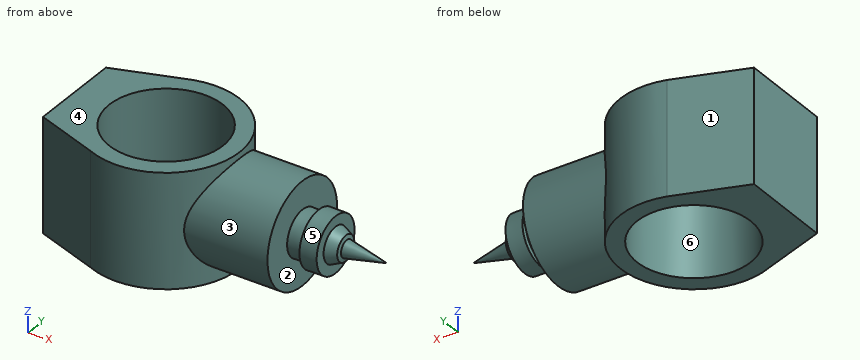
```python
from build123d import *

# Parameters (mm, degrees)
SKETCH1_R                = 50
BOSS_EXTRUDE1_DEPTH      = 50
BOSS_EXTRUDE2_REACH      = 218.485
BOSS_EXTRUDE2_END_RADIUS = 65
SKETCH2_R                = 45


with BuildPart() as part:
    # Sketch1 → Boss-Extrude1 (new, symmetric)
    with BuildSketch(Plane.XY):
        with BuildLine():
            Line((-80.332774103, 40.816671374), (-18.32732241, 62.420380787))
            ThreePointArc((-18.32732241, 62.420380787), (64.887320327, -3.869658553), (-25.718765207, -59.633296758))
            Line((-25.718765207, -59.633296758), (-80.331207523, -40.594442176))
            Line((-80.331207523, -40.594442176), (-80.332774103, 40.816671374))
        make_face()
        with Locations(Location((0.059475093, 0.33297887, 0), (0, 0, 180))):
            Circle(SKETCH1_R, mode=Mode.SUBTRACT)
    extrude(amount=BOSS_EXTRUDE1_DEPTH, both=True)

    # Boss-Extrude2: up to this cylinder (the profile starts outside it)
    boss_extrude2_end = Plane(origin=(0.006183555, 0.059475093, -0.380635), z_dir=(0, 0, -1)) * Cylinder(BOSS_EXTRUDE2_END_RADIUS, 567.97, mode=Mode.PRIVATE)
    # Sketch2 → Boss-Extrude2 (add, up to the surface)
    with BuildSketch(Plane(origin=(120, 0, 0), x_dir=(0, 0, -1), z_dir=(1, 0, 0)), mode=Mode.PRIVATE) as boss_extrude2_sk1:
        with Locations((0.380634668, -0.130842241)):
            Circle(SKETCH2_R)
    boss_extrude2_tool1 = extrude(boss_extrude2_sk1.sketch, amount=-BOSS_EXTRUDE2_REACH, mode=Mode.PRIVATE) - boss_extrude2_end
    add(boss_extrude2_tool1.solids().sort_by_distance((120, -0.130842, -0.380635))[0])

    # Sketch4 → Revolve1 (revolve)
    with BuildSketch(Plane.XY):
        Polygon((119.999333132, 0.283284997), (194.173107585, 0.294264183), (158.779171315, -7.089790216), (157.928859049, -10.799864107), (148.89148066, -15.080727554), (148.998076603, -24.232348433), (133.998076603, -24.369382261), (133.994271745, -19.369382261), (119.994271745, -19.700497331), align=None)
    revolve(axis=Axis((119.999333132, 0.283284997, 0), (0.9999999890450703, 0.00014801979444003187, 0)))


solid = part.part
```
The listing builds one solid part. Answer for the finished solid, in the listing's coordinates (mm). Face numbers are marked on the shaded views. A direction names the side the tool comes from. Round coordinates to 2 decimals unless told otherwise and drop trailing zeros. Order: outer loops, then holes, each group sorted by start corner. A loop starts at its lowest first (then second) coordinate and runs counter-clockwise, first axis right, second up. Notation, with made-up numbers: (61.25, 32.25) -> (65.25, 32.25) arc R20 ccw to (65.25, 64.25) -> close; hole circle Ø7 at (-13.5, 15.25). An arc over 180 degrees is marked (long way). Answer as CSV lines item,"result".
Q1. Consider line 1 (X direction, y = 0, z = 17); line 2 (Y direction, x = -36.5, z = 5); line 3 (X direction, y = 11.5, z = 43). Determine where each line is inside the solid, lowest interval first. Write a range as from..to.
Computed values:
line 1,"x = -80.33..-49.94, 50.06..148.91"
line 2,"y = -55.87..-33.78, 34.44..56.09"
line 3,"x = -80.33..-48.68, 48.8..120"
Q2. For a pull along Y with two mould halves and no side action, classify the marked faces 4, 5 and 6 as +Y half, -Y half, draft (parallel to the pull), parting line (faces both ways), or undercut.
Computed values:
face 4,"draft"
face 5,"parting line"
face 6,"undercut"
Q3. A cutting plane is placed at B-B on z = 40.5. Determine the outline of the cut face in (x, y), plus the area to 3 significant figures.
Computed values:
outline,"(-80.33, -40.59) -> (-25.72, -59.63) arc R65 ccw to (62.17, -18.94) -> (120, -18.94) -> (120, 18.68) -> (62.28, 18.68) arc R65 ccw to (-18.33, 62.42) -> (-80.33, 40.82) -> close; hole circle Ø100 at (0.06, 0.33)"
area,"9,630 mm^2"
Q4. Given pin 1 (8 mm diameter, centred on x = 112.5, y = 5, fed in from +Z); pin 2 (1 mm diameter, centred on x = 52, z = 6.5, fed in from +Y), each flat-ended and moving along its own axis, determine where each tip first touches the part or whether it passes through.
Computed values:
pin 1,"stops at z = 44.61"
pin 2,"stops at y = 44.41"
Q5. Which of the six approach directions +Z, -Z, +X, -X, +Y, -Y give full straight-line access (tool end or side, diameter ignored) to the marked faces 1, 2 and 3?
Computed values:
face 1,"+Z, -Z, -X, +Y"
face 2,"none"
face 3,"+X"
Q6. A cutting plane is placed at A-A on x = 8.5. Determine the outline of the cut face in (y, z), plus the area to 3 significant figures.
Computed values:
outline,"(-64.38, -50) -> (-48.95, -50) -> (-48.95, 50) -> (-64.38, 50) -> close; (49.62, -50) -> (64.5, -50) -> (64.5, 50) -> (49.62, 50) -> close"
area,"3,030 mm^2"
Q7. A cutting plane is placed at D-D on x = 107. Determine the outline of the cut face in (y, z).
Computed values:
outline,"circle Ø90 at (-0.13, -0.38)"
Q8. A cutting plane is placed at C-C on z = -37. Determine the outline of the cut face in (x, y), plus the area to 3 significant figures.
Computed values:
outline,"(-80.33, -40.59) -> (-25.72, -59.63) arc R65 ccw to (59.43, -26.28) -> (120, -26.28) -> (120, 26.02) -> (59.6, 26.02) arc R65 ccw to (-18.33, 62.42) -> (-80.33, 40.82) -> close; hole circle Ø100 at (0.06, 0.33)"
area,"10,500 mm^2"
